Answer from the drawing. Dimensions are ordinates in mm from the lowest x, y and z of the part. A direction names the side the tool comes from. Coordinates: 2 decimals unless noted, no trailing zeros. Loops run counter-clockwise (first coordinate to the right, second up) from the corner with the lowest first, then second, coordinate; pieces in that order, holes last. Notation, with made-up numbers: (18, -4) - (77, -4) arc R29 cw to (77, 20) - close; hole circle Ø7 at (-9.75, 75.5). An arc over 180 degrees is marked (long way). Write each question's results on one line, items separated by ' | '. Start each with the question number.
1. A cutting plane is placed at A-A on z = 15. Determine the outline of the cut face in (x, y), then the cut area to 3 significant figures.
2. Which of the six approach directions +Z, -Z, +X, -X, +Y, -Y give full straight-line access (tool end or side, diameter ignored) to the marked faces 1 and 2?
3. A cutting plane is placed at B-B on y = 7. Determine the outline of the cut face in (x, z), then the cut area to 3 significant figures.
4. Find the intervals of material crossed by line 1 along Y through (x, z) = (20.5, 4.75); line 2 along X through (y, z) = (46.5, 15.5), in increasing order. Write a range as [from, to].
5. Each of these flat-tipped pins is pushed along its axis until it touches: P1, Ø8, axis at y = 44.5, z = 12.5, coming from the -X side; P2, Ø4, axis at y = 20.5, z = 23, coming from the +X side; P3, Ø4, axis at x = 15.05, y = 7, coming from the +Z side. Where does it stop, or does it pass through?
6. A cutting plane is placed at C-C on y = 17.5. Determine the outline of the cut face in (x, z).
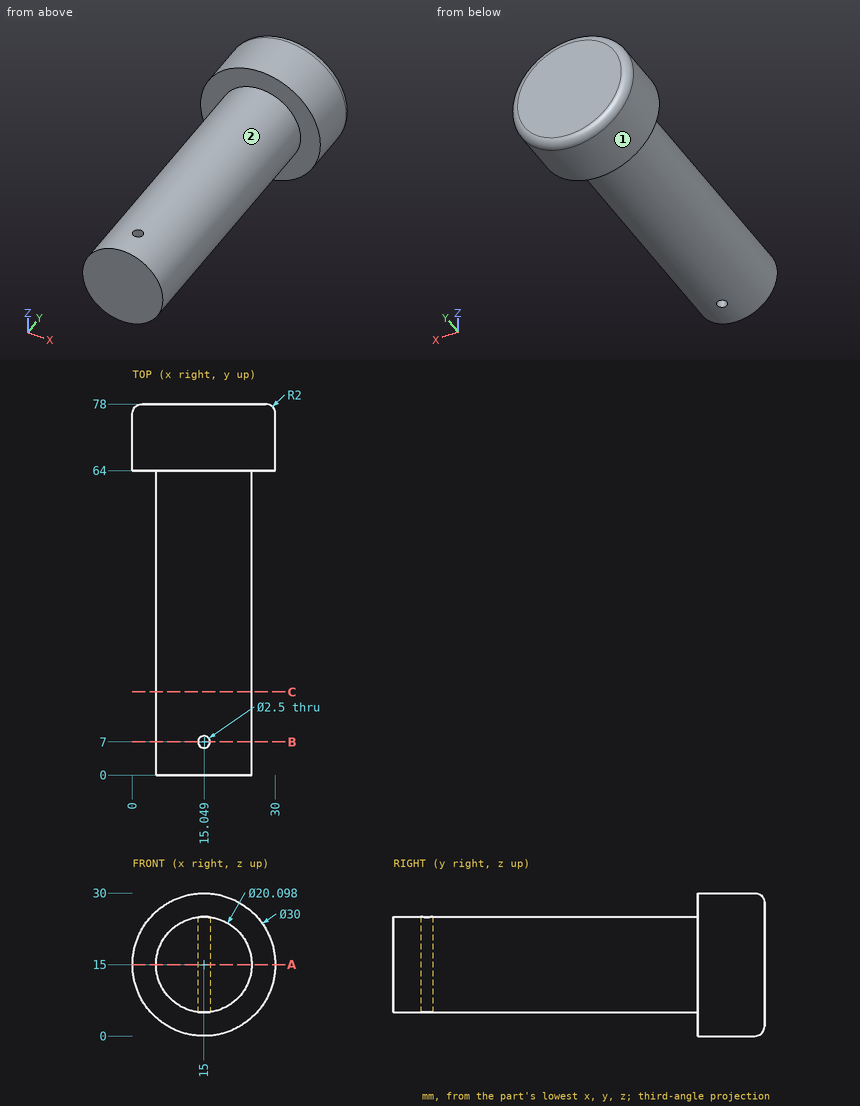
Values:
1) outline: (0, 64) - (4.95, 64) - (4.95, 0) - (25.05, 0) - (25.05, 64) - (30, 64) - (30, 76) arc R2 ccw to (28, 78) - (2, 78) arc R2 ccw to (0, 76) - close; hole circle Ø2.5 at (15.05, 7) | area: 1,700 mm^2
2) face 1: +Y, -Y | face 2: -Y
3) outline: (13.8, 5.02) - (13.8, 24.98) arc R10.05 ccw to start; (16.3, 5.04) arc R10.05 ccw to (16.3, 24.96) - close | area: 267 mm^2
4) line 1: [64, 78] | line 2: [4.96, 25.04]
5) P1: x = 4.95 | P2: x = 23.06 | P3: z = 25.05
6) outline: circle Ø20.1 at (15, 15)
